Source: CAD feature listing. Evaluate the final solid. Frame: model axes, mm. A direction names the side the tool comes from. Give positions to 0.01 mm unless a question says otherwise; leave off trailing zeros. Order: outer loops, then holes, each group sorted by start corner. A loop starts at its lowest first (then second) coordinate and runs counter-clockwise, first axis right, second up. Notation, with made-up numbers: M 77.5,88.25 L 99.5,88.25 A28 ccw 99.5,118.25 Z; hole C 32,77.25 d3. An arc over 180 degrees is marked long. Answer as a JSON object with one key per item and string values. Group by question number.
1. Pin query (flat end, axial travel): P1, Ø23, axis at x = -8, z = 24, coming from the -Y side; P2, Ø23, axis at x = -13.5, y = -28.5, coming from the +Z side; P3, Ø5, axis at x = 17.5, z = 39.5, coming from the +Y side; P4, Ø17, axis at x = -10.5, z = 17, coming from the +Y side. Return the tip coordinate at first contact, or that it passes through.
2. Section query D-D (z = 32). Output: boundary loops of the cut face in (x, y), plus the area to 3 significant figures.
3. Material intervals for L1, parallel to Y at x = 45, z = 44.5; L2, parallel to X at y = -11, z = 9.5; L3, parallel to Y at x = -14, z = 12.5, sorted ascending. Write a range as [from, to].
4. Set-up query: faces 1 (the flat face through (-10, -13.937, 21)), 2 (the flat face through (-10, -27, 33.99)), 3 (the flat face through (25, -50.8, 37)). Return all of +Z, -Z, +X, -X, +Y, -Y with unobstructed straight access to the full face (end or side cutting, diameter ignored); none if empty.
5. Section query A-A (y = -34). Output: boundary loops of the cut face in (x, z).
6. Section query B-B (z = 20). Output: boundary loops of the cut face in (x, y).
7. Section query C-C (x = 33.5). Output: boundary loops of the cut face in (y, z), plus the area to 3 significant figures.
from build123d import *

# Parameters (mm, degrees)
F0_W     = 50.8
F0_H     = 50.8
F1_DEPTH = 50.8
F2_R     = 12.7
F3_DEPTH = 63.5
F4_W     = 25.4
F4_H     = 25.4
F5_DEPTH = 21.082


with BuildPart() as f1:
    # F0 (on Front) → F1 (new body)
    with BuildSketch(Plane.XZ):
        with Locations((25.4, 25.4)):
            Rectangle(F0_W, F0_H)
    extrude(amount=F1_DEPTH)

    # F2 (on Front) → F3 (join)
    with BuildSketch(Plane.XZ):
        with Locations((24.060287, 23.105513)):
            Circle(F2_R)
    extrude(amount=F3_DEPTH)

    # F4 (on Right) → F5 (join)
    with BuildSketch(Plane.YZ):
        with Locations((-26.636659, 21.289929)):
            Rectangle(F4_W, F4_H)
    extrude(amount=-F5_DEPTH)


solid = f1.part
Answer sheet:
{
 "1": {"P1": "y = -50.8", "P2": "z = 33.99", "P3": "y = 0", "P4": "y = -13.94"},
 "2": {"outline": "M -21.08,-39.34 L 0,-39.34 L 0,-50.8 L 15,-50.8 L 15,-63.5 L 33.13,-63.5 L 33.13,-50.8 L 50.8,-50.8 L 50.8,0 L 0,0 L 0,-13.94 L -21.08,-13.94 Z", "area": "3,350 mm^2"},
 "3": {"L1": "[-50.8, 0]", "L2": "[0, 50.8]", "L3": "[-39.34, -13.94]"},
 "4": {"face 1": "+Z, -Z, -X, +Y", "face 2": "+Z, -X, +Y, -Y", "face 3": "-Y"},
 "5": {"outline": "M -21.08,8.59 L 0,8.59 L 0,0 L 50.8,0 L 50.8,50.8 L 0,50.8 L 0,33.99 L -21.08,33.99 Z"},
 "6": {"outline": "M -21.08,-39.34 L 0,-39.34 L 0,-50.8 L 11.75,-50.8 L 11.75,-63.5 L 36.37,-63.5 L 36.37,-50.8 L 50.8,-50.8 L 50.8,0 L 0,0 L 0,-13.94 L -21.08,-13.94 Z"},
 "7": {"outline": "M -63.5,14.61 L -50.8,14.61 L -50.8,0 L 0,0 L 0,50.8 L -50.8,50.8 L -50.8,31.6 L -63.5,31.6 Z", "area": "2,800 mm^2"}
}
